For this review, take the finished solid that the model builds, in its own axes (mm). Face numbers are marked on the shaded views. A direction names the side the tool comes from. Give positions to 0.01 mm unless a question says otherwise; leave off trailing zeros. Order: outer loops, then holes, each group sorted by start corner. A loop starts at its lowest first (then second) coordinate and runs counter-clockwise, first axis right, second up. Notation, with made-up numbers: M 42.5,56.25 L 63.5,56.25 A24 cw 63.5,66.25 Z; hole C 36,40.5 d6. An arc over 180 degrees is marked long. Use CSV: the item, a comma, the result in double quotes. Start each with the question number.
(1) Consider section C-C (y = 9.5). Give the number of separate pieces and of enclosed holes in the cut face, and give its area (3 significant figures).
(2) Draft analysis for pull direction Z (two halves, no side actions). For the marked faces 3, 4, 5 and 6, state which applies: pulls with the +Z half, pulls with the -Z half, needs draft (parallel to the pull), parting line crosses it, or undercut.
(3) Clearance check with flat-ended pins moving along their axes: P1, Ø2, axis at x = -11, y = 10.5, coming from the +Z side; P2, Ø4.5, axis at x = -3, z = -20, coming from the +Y side; P3, Ø1.5, axis at y = 12.5, z = -24, coming from the -X side; P4, Ø16.5, axis at x = 2.5, z = 19.5, coming from the +Y side. State where each tip first meets the part, or that it passes through.
(4) Consider section A-A (z = 0). Write out the cut boundary in (x, y), and give its area (3 significant figures).
(5) Wall thickness on L1, parallel to X at y = 5, z = 0; L2, parallel to Z at x = 13, y = 7.25; L3, parallel to Z at x = 5, y = 9.5 (3 decimals): over which ranges is each line inside the solid? List them lowest first. Write a range as from..to.
(6) Tool access review of the marked faces 1 and 2: name each direction out of +Z, -Z, +X, -X, +Y, -Y from which nothing blocks a thin tool from reaching the whole face with its end or side.
(7) Consider section B-B (x = 0). Write out the cut boundary in (y, z).
(8) Consider section D-D (x = -17.5). Write out the cut boundary in (y, z), and give its area (3 significant figures).
```python
from build123d import *

# Parameters (mm, degrees)
SKETCH1_R             = 57.5
BOSS_EXTRUDE1_DEPTH   = 16
SKETCH2_R             = 12.5
CUT_EXTRUDE1_DEPTH    = 83.876414015
SKETCH3_R             = 7.439291055
CUT_EXTRUDE2_DEPTH    = 12.432983
CIRPATTERN1_START     = 3.567017068
CIRPATTERN1_OUTLINE_R = 7.439291055
CIRPATTERN1_DEPTH     = 12.432982932


# Read off the part's stored shape, not the designer's step: CirPattern1
with BuildPart() as part:
    # Sketch1 → Boss-Extrude1 (new body)
    with BuildSketch(Plane(origin=(0, 0, 0), x_dir=(1, 0, 0), z_dir=(0, 1, 0))):
        with Locations(Location((0, 0, 0), (0, 0, 270))):
            Circle(SKETCH1_R)
    extrude(amount=BOSS_EXTRUDE1_DEPTH)

    # Sketch2 → Cut-Extrude1 (cut, through all)
    with BuildSketch(Plane(origin=(0, 0, 0), x_dir=(1, 0, 0), z_dir=(0, 1, 0))):
        with Locations(Location((0, 0, 0), (0, 0, 270))):
            Circle(SKETCH2_R)
    extrude(amount=CUT_EXTRUDE1_DEPTH, mode=Mode.SUBTRACT)

    # Sketch3 → Cut-Extrude2 (cut)
    with BuildSketch(Plane(origin=(0, 16, 0), x_dir=(1, 0, 0), z_dir=(0, 1, 0))):
        with Locations(Location((-21.336549902, 0, 0), (0, 0, 270))):
            Circle(SKETCH3_R)
    extrude(amount=-CUT_EXTRUDE2_DEPTH, mode=Mode.SUBTRACT)

    # CirPattern1 outline → CirPattern1 (cut)
    with BuildSketch(Plane(origin=(0, 0, 0), x_dir=(1, 0, 0), z_dir=(0, 1, 0)).offset(CIRPATTERN1_START)):
        with Locations((-15.087219123, -15.087219123)):
            Circle(CIRPATTERN1_OUTLINE_R)
        with Locations((-15.087219123, 15.087219123)):
            Circle(CIRPATTERN1_OUTLINE_R)
        with Locations((0, 21.336549902)):
            Circle(CIRPATTERN1_OUTLINE_R)
        with Locations((15.087219123, 15.087219123)):
            Circle(CIRPATTERN1_OUTLINE_R)
        with Locations((21.336549902, 0)):
            Circle(CIRPATTERN1_OUTLINE_R)
        with Locations((15.087219123, -15.087219123)):
            Circle(CIRPATTERN1_OUTLINE_R)
        with Locations((0, -21.336549902)):
            Circle(CIRPATTERN1_OUTLINE_R)
    extrude(amount=CIRPATTERN1_DEPTH, mode=Mode.SUBTRACT)


solid = part.part
```
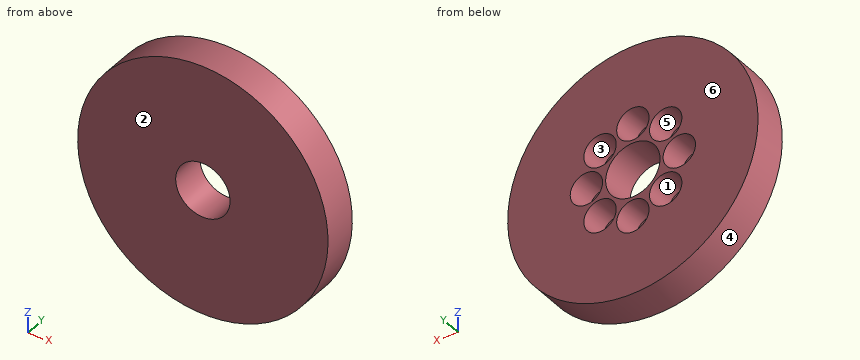
Check result:
1,separate pieces,"1"
1,enclosed holes,"9"
1,area,"8,510 mm^2"
2,face 3,"undercut"
2,face 4,"parting line crosses it"
2,face 5,"undercut"
2,face 6,"needs draft"
3,P1,"stops at z = 56.62"
3,P2,"stops at y = 3.57"
3,P3,"stops at x = -52.59"
3,P4,"stops at y = 16"
4,outline,"M -57.5,0 L -12.5,0 L -12.5,16 L -13.9,16 L -13.9,3.57 L -28.78,3.57 L -28.78,16 L -57.5,16 Z; M 12.5,0 L 57.5,0 L 57.5,16 L 28.78,16 L 28.78,3.57 L 13.9,3.57 L 13.9,16 L 12.5,16 Z"
4,area,"1,070 mm^2"
5,L1,"x = -57.5..-28.78, -13.9..-12.5, 12.5..13.9, 28.78..57.5"
5,L2,"z = -56.01..-22.23, -7.95..7.95, 22.23..56.01"
5,L3,"z = -57.282..-26.845, -15.828..-11.456, 11.456..15.828, 26.845..57.282"
6,face 1,"+Y"
6,face 2,"+Z, -Z, +X, -X, -Y"
7,outline,"M 0,-57.5 L 16,-57.5 L 16,-28.78 L 3.57,-28.78 L 3.57,-13.9 L 16,-13.9 L 16,-12.5 L 0,-12.5 Z; M 0,12.5 L 16,12.5 L 16,13.9 L 3.57,13.9 L 3.57,28.78 L 16,28.78 L 16,57.5 L 0,57.5 Z"
8,outline,"M 0,-54.77 L 16,-54.77 L 16,-22.12 L 3.57,-22.12 L 3.57,-8.05 L 16,-8.05 L 16,-6.37 L 3.57,-6.37 L 3.57,6.37 L 16,6.37 L 16,8.05 L 3.57,8.05 L 3.57,22.12 L 16,22.12 L 16,54.77 L 0,54.77 Z"
8,area,"1,240 mm^2"
